The figure shows three views and two pictorial views of one solid part (mm, origin at its lowest corner). Answer the questions. Give positions to 0.01 mm unless a question says otherwise; leave off trailing zeros. Write each loop counter-clockwise with the first axis right and the second up, starting at its lowest first coordinate (ties: lowest second). Pieces come first, ordered by that corner, then holes. Notation, with made-up numbers: (76, -22.75) - (104, -22.75) arc R31 cw to (104, 14.25) - close; hole circle Ø8 at (-36.75, 75). An arc over 180 degrees is marked (long way). One line per question, with ' | ' between items. Start each with the question number.
1. Given P1, Ø10, axis at y = 5, z = 289.5, coming from the -X side; P2, Ø1, axis at x = 2, y = 12, coming from the +Z side; P3, Ø5, axis at x = 1.5, z = 152, coming from the +Y side (1 decimal), each flat-ended and moving along its own axis, determine where each tip first touches the part or whether it passes through.
2. Find the intervals of material crossed by L1, parallel to Z at x = 12.75, y = 5.5; L2, parallel to X at y = 25, z = 89; L3, parallel to X at y = 11, z = 62.5, in increasing order. Write a range as from..to.
3. A cutting plane is placed at A-A (x = 8). Determine the outline of the cut face in (y, z).
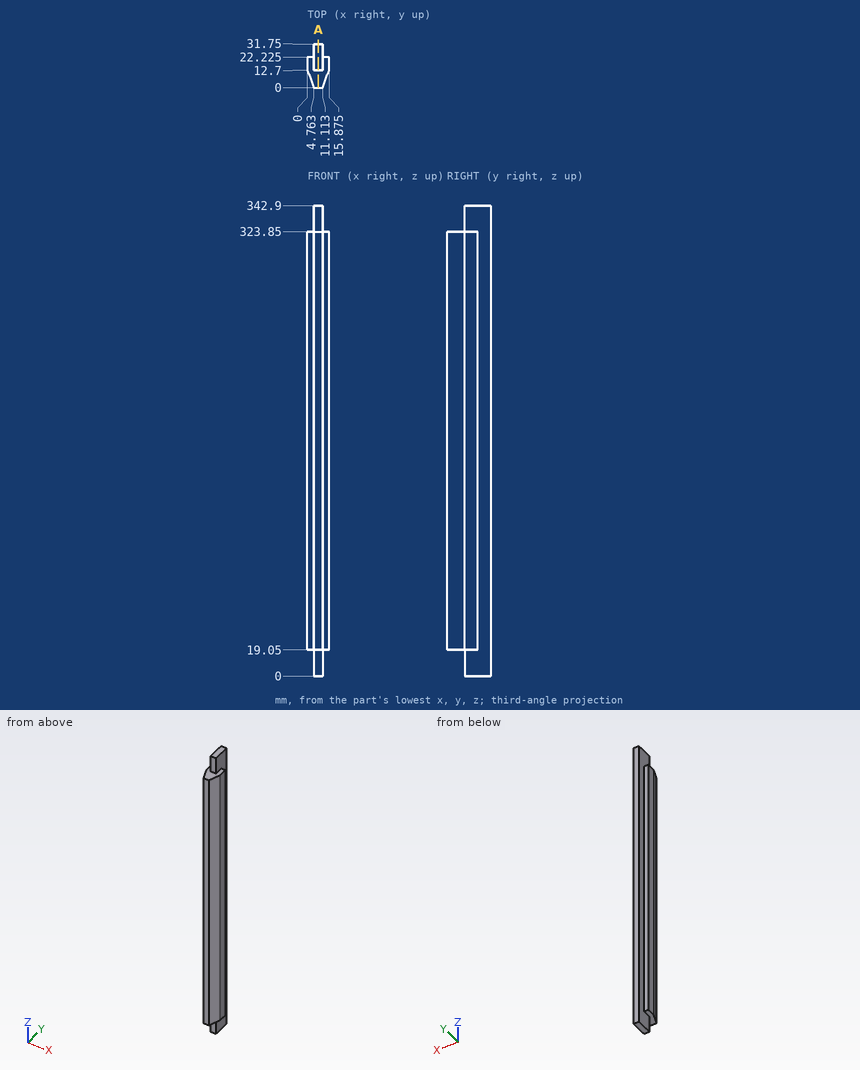
Determined:
1) P1: x = 1.01 | P2: z = 323.85 | P3: y = 22.2
2) L1: 19.05..323.85 | L2: 4.76..11.11 | L3: 0.64..15.24
3) outline: (0, 19.05) - (12.7, 19.05) - (12.7, 0) - (31.75, 0) - (31.75, 342.9) - (12.7, 342.9) - (12.7, 323.85) - (0, 323.85) - close
